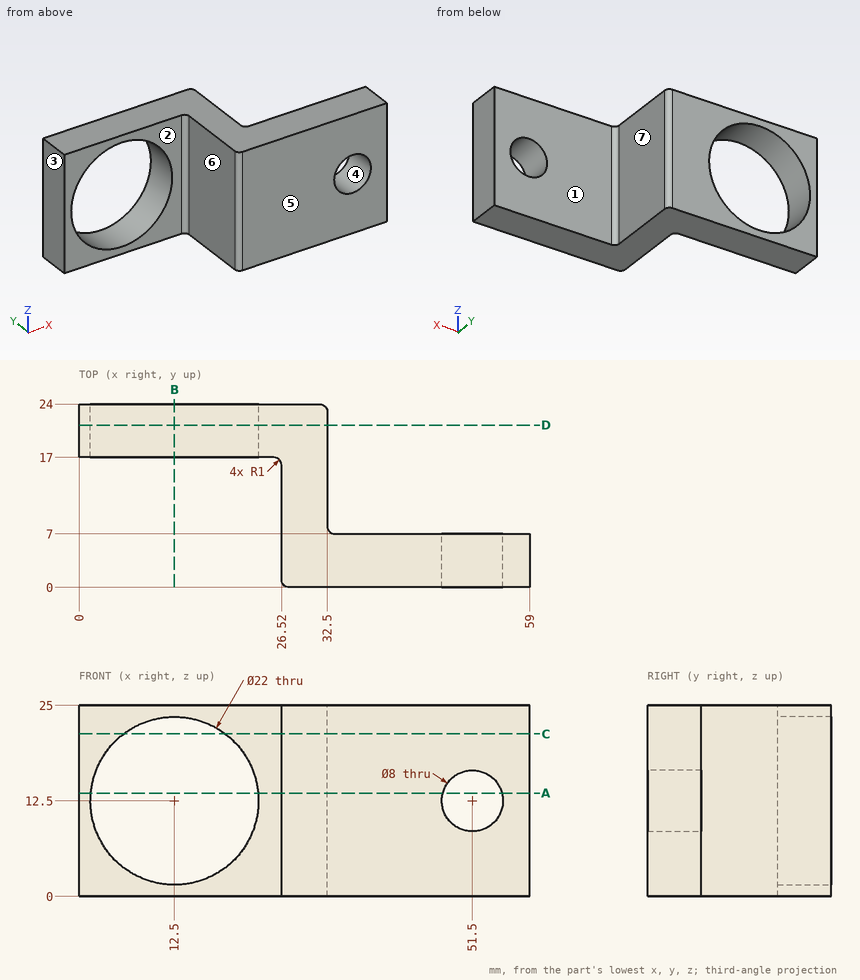
Drawing for the job (mm, zero at the part's lowest x, y, z). A direction names the side the tool comes from. Round coordinates to 2 decimals unless told otherwise and drop trailing zeros. Loops run counter-clockwise (first coordinate to the right, second up) from the corner with the lowest first, then second, coordinate; pieces in that order, holes last. Notation, with made-up numbers: (22, -22.75) - (28, -22.75) arc R11 cw to (28, -16.75) - close; hole circle Ø11 at (75.5, 67). An arc over 180 degrees is marked (long way). Return JSON: item names as keys, results as strings. Group by question number.
Q1. Band-saw the part on A-A on z = 13.5. Give the cut face in (x, y), plus the area to 3 significant figures.
Q2. Tool access for the marked faces 1, 2 and 3: list every direction of +Z, -Z, +X, -X, +Y, -Y with a clear straight run to the whole face (end or side of a thin tool).
Q3. Band-saw the part on B-B on x = 12.5. Give the cut face in (y, z).
Q4. Two-plate mould, pull along X, no slides. Class the marked faces 4, 5, 6 and 7: +X half, -X half, draft (parallel to the pull), parting line (faces both ways), or undercut.
Q5. Band-saw the part on D-D on y = 21.25. Give the cut face in (x, z).
Q6. Flat gauge pins, fed straight in: pin 1 Ø12 at (y, z) = (5, 13.5) entering from -X; pin 2 Ø4.5 at (y, z) = (12, 15) entering from +X; pin 3 Ø9 at (x, z) = (51.5, 12.5) entering from +Y; pin 4 Ø1 at (x, y) = (14.5, 15) entering from +Z. Where does each tip first touch, or does it go through?
Q7. Drill centre lines: line 1 along X through (y, z) = (3.5, 12.5); line 2 along X through (y, z) = (21, 12.5); line 3 along X through (y, z) = (14.75, 21.25). Where is each one in solid material? Low to high. Write a range as [from, to].
Q8. Band-saw the part on C-C on z = 21.25. Give the cut face in (x, y).
Solutions:
{
 "1": {"outline": "(0, 17) - (1.55, 17) - (1.55, 24) - (0, 24) - close; (23.45, 17) - (25.52, 17) arc R1 cw to (26.52, 16) - (26.52, 1) arc R1 ccw to (27.52, 0) - (47.63, 0) - (47.63, 7) - (33.5, 7) arc R1 cw to (32.5, 8) - (32.5, 23) arc R1 ccw to (31.5, 24) - (23.45, 24) - close; (55.37, 0) - (59, 0) - (59, 7) - (55.37, 7) - close", "area": "307 mm^2"},
 "2": {"face 1": "+Z, -Z, +X, +Y", "face 2": "+Z, -Z, -X, -Y", "face 3": "+Z, -Z, -X, +Y, -Y"},
 "3": {"outline": "(17, 0) - (24, 0) - (24, 1.5) - (17, 1.5) - close; (17, 23.5) - (24, 23.5) - (24, 25) - (17, 25) - close"},
 "4": {"face 4": "undercut", "face 5": "draft", "face 6": "-X half", "face 7": "+X half"},
 "5": {"outline": "(0, 0) - (32.5, 0) - (32.5, 25) - (0, 25) - close; hole circle Ø22 at (12.5, 12.5)"},
 "6": {"pin 1": "stops at x = 26.52", "pin 2": "stops at x = 32.5", "pin 3": "stops at y = 7", "pin 4": "passes through"},
 "7": {"line 1": "x = [26.52, 47.5], [55.5, 59]", "line 2": "x = [0, 1.5], [23.5, 32.5]", "line 3": "x = [26.52, 32.5]"},
 "8": {"outline": "(0, 17) - (5.83, 17) - (5.83, 24) - (0, 24) - close; (19.17, 17) - (25.52, 17) arc R1 cw to (26.52, 16) - (26.52, 1) arc R1 ccw to (27.52, 0) - (59, 0) - (59, 7) - (33.5, 7) arc R1 cw to (32.5, 8) - (32.5, 23) arc R1 ccw to (31.5, 24) - (19.17, 24) - close"}
}
